The figure shows three views and two pictorial views of one solid part (mm, origin at its lowest corner). Answer the questions. A direction names the side the tool comes from. Round coordinates to 2 decimals unless told otherwise and drop trailing zeros. Order: outer loops, then holes, each group sorted by start corner. A loop starts at its lowest first (then second) coordinate and runs counter-clockwise, first axis right, second up. Notation, with made-up numbers: (-25.75, 73) - (8.25, 73) arc R19 cw to (8.25, 109) - close; hole circle Ø8 at (50, 1.5). An arc over 180 degrees is marked (long way). One line per item, written item: value. Start each with the question number.
1. Straight lines are drawn through the part: line 1 (X direction, y = 2, z = 20); line 2 (Z direction, x = 34.5, y = 7.5); line 3 (Z direction, x = 18, y = 7.75) (1 decimal). For each, find the intervals that lie inside material, in ascending order.
2. Section B-B, the plane x = 35 is taken. Give the vertices of the cut face in (y, z), then the cut area to 3 significant figures.
3. A tool of negligible diameter and unlimited length cuts with its end or side. For the marked faces 1 and 2, from which of +Z, -Z, +X, -X, +Y, -Y can it reach the whole face along a straight path? Write none if from no direction.
4. For a pull along Z with two mould halves and no side action, classify the marked faces 3, 4 and 5 as released by +Z, released by -Z, zero draft, split by the parting line, or undercut.
5. A flat-ended cylindrical pin translates along its axis: P1, Ø4, axis at x = 35.5, z = 19.5, coming from the +Y side. Find the tip coordinate at first contact, or state that the pin passes through.
6. Section C-C, the plane y = 17 is taken. Give the vertices of the cut face in (x, z) (1 decimal).
7. Section A-A, the plane z = 6 is taken. Give the vertices of the cut face in (x, y).
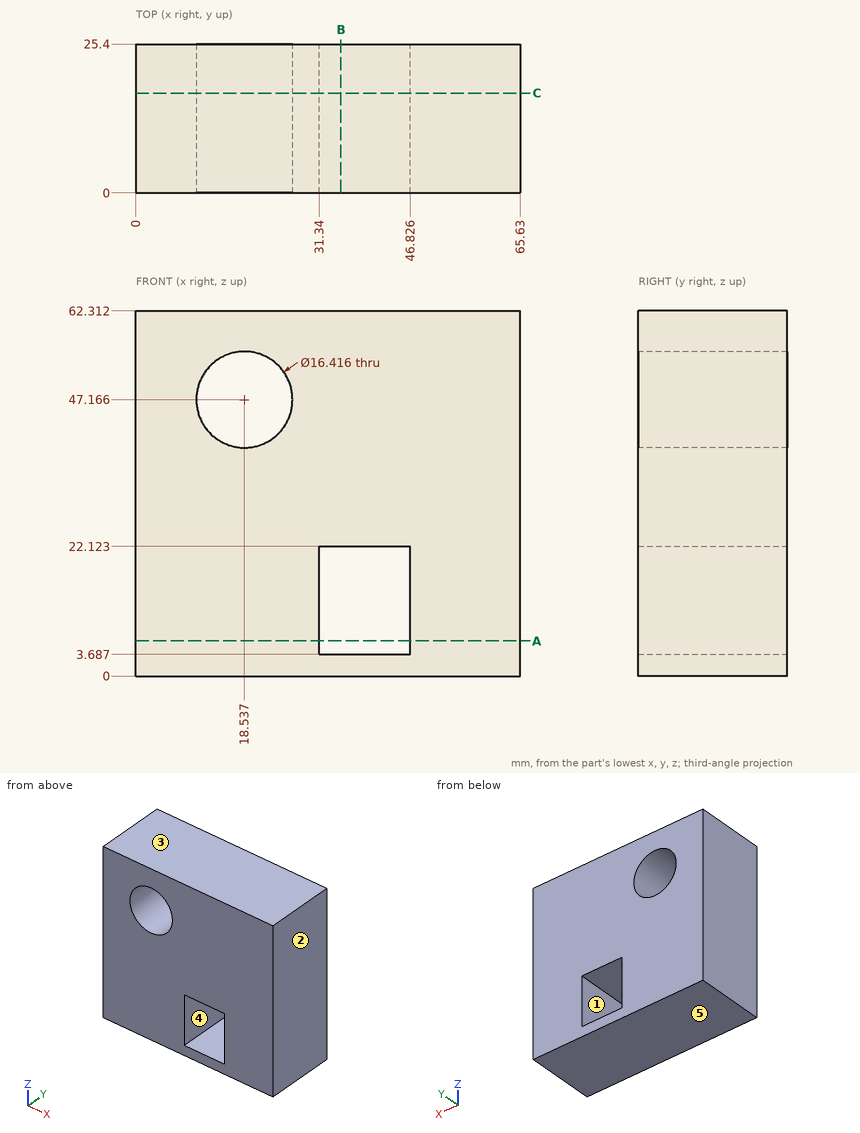
Answer list:
1. line 1: x = 0 to 31.34, 46.83 to 65.63
1. line 2: z = 0 to 3.69, 22.12 to 62.31
1. line 3: z = 0 to 39, 55.4 to 62.3
2. outline: (0, 0) - (25.4, 0) - (25.4, 3.69) - (0, 3.69) - close; (0, 22.12) - (25.4, 22.12) - (25.4, 62.31) - (0, 62.31) - close
2. area: 1,110 mm²
3. face 1: +Y, -Y
3. face 2: +Z, -Z, +X, +Y, -Y
4. face 3: released by +Z
4. face 4: undercut
4. face 5: released by -Z
5. P1: passes through
6. outline: (0, 0) - (65.6, 0) - (65.6, 62.3) - (0, 62.3) - close; hole circle Ø16.4 at (18.5, 47.2); hole (31.3, 3.7) - (46.8, 3.7) - (46.8, 22.1) - (31.3, 22.1) - close
7. outline: (0, 0) - (31.34, 0) - (31.34, 25.4) - (0, 25.4) - close; (46.83, 0) - (65.63, 0) - (65.63, 25.4) - (46.83, 25.4) - close
